Read the model definition and answer for the solid it produces. Units are mm, in the model's axes. Face numbers are marked on the shaded views. A direction names the side the tool comes from. Give positions to 0.01 mm unless a question says otherwise; leave off trailing zeros. Write each loop counter-clockwise with the first axis right and the second up, starting at its lowest first coordinate (ties: lowest second). Pieces come first, ordered by that corner, then holes.
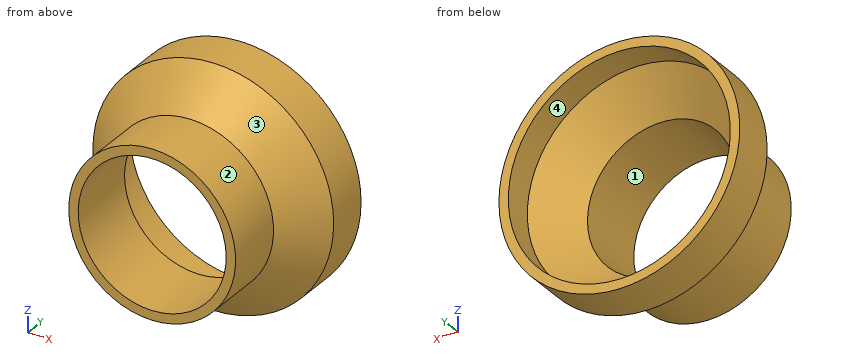
```python
from build123d import *

# Parameters (mm, degrees)
SKETCH1_R           = 15.748
SKETCH1_R_2         = 13.97
BOSS_EXTRUDE1_DEPTH = 19.05
SKETCH2_R           = 22.733
SKETCH2_R_2         = 13.97
BOSS_EXTRUDE2_DEPTH = 7.62
SKETCH3_R           = 20.955
CUT_EXTRUDE1_DEPTH  = 5.08
CHAMFER1_SIZE       = 7.62
CHAMFER2_SIZE       = 7.62


with BuildPart() as part:
    # Sketch1 → Boss-Extrude1 (new body)
    with BuildSketch(Plane(origin=(0, 0, 0), x_dir=(1, 0, 0), z_dir=(0, 1, 0))):
        with Locations(Location((0, 0, 0), (0, 0, 90))):
            Circle(SKETCH1_R)
        with Locations(Location((0, 0, 0), (0, 0, 90))):
            Circle(SKETCH1_R_2, mode=Mode.SUBTRACT)
    extrude(amount=BOSS_EXTRUDE1_DEPTH)

    # Sketch2 → Boss-Extrude2 (add)
    with BuildSketch(Plane(origin=(0, 19.05, 0), x_dir=(1, 0, 0), z_dir=(0, 1, 0))):
        with Locations(Location((0, 0, 0), (0, 0, 90))):
            Circle(SKETCH2_R)
        with Locations(Location((0, 0, 0), (0, 0, 90))):
            Circle(SKETCH2_R_2, mode=Mode.SUBTRACT)
    extrude(amount=BOSS_EXTRUDE2_DEPTH)

    # Sketch3 → Cut-Extrude1 (cut)
    with BuildSketch(Plane(origin=(0, 26.67, 0), x_dir=(1, 0, 0), z_dir=(0, 1, 0))):
        with Locations(Location((0, 0, 0), (0, 0, 270))):
            Circle(SKETCH3_R)
    extrude(amount=-CUT_EXTRUDE1_DEPTH, mode=Mode.SUBTRACT)

    # Chamfer1
    # the kernel refuses this chamfer: 7.62 mm, written as the material it adds along each edge
    with BuildSketch(Plane(origin=(0, 19.05, 0), x_dir=(0, 0, -1), z_dir=(1, 0, 0))) as chamfer1_piece_1_section:
        Polygon((15.748, -CHAMFER1_SIZE), (15.748 + CHAMFER1_SIZE, 0), (15.748, 0), align=None)
    chamfer1_piece_1 = revolve(axis=Axis((0, 19.05, 0), (0, 1, 0)), mode=Mode.PRIVATE)
    chamfer1_piece_1 = chamfer1_piece_1 & Plane(origin=(0, 14.923095596, 0), x_dir=(0, 0, -1), z_dir=(0, -1, 0)) * Cylinder(22.733, 94, mode=Mode.PRIVATE)
    add(chamfer1_piece_1)

    # Chamfer2
    # the kernel refuses this chamfer: 7.62 mm, written as the material it takes off along each edge
    with BuildSketch(Plane(origin=(0, 21.59, 0), x_dir=(0, 0, -1), z_dir=(-1, 0, 0))) as chamfer2_piece_1_section:
        Polygon((13.97, CHAMFER2_SIZE), (13.97 + CHAMFER2_SIZE, 0), (13.97, 0), align=None)
    chamfer2_piece_1 = revolve(axis=Axis((0, 21.59, 0), (0, -1, 0)), mode=Mode.PRIVATE)
    chamfer2_piece_1 = chamfer2_piece_1 & Plane(origin=(0, 17.459443448, 0), x_dir=(0, 0, 1), z_dir=(0, 1, 0)) * Cylinder(20.955, 87, mode=Mode.PRIVATE)
    add(chamfer2_piece_1, mode=Mode.SUBTRACT)


solid = part.part
```
Item 1: Determine the mould class of the marked faces 1 and 2 for opening direction Z: pulls with the +Z half, pulls with the -Z half, needs draft (parallel to the pull), parting line crosses it, or undercut.
Result set:
face 1: undercut
face 2: parting line crosses it
Item 2: Each of these flat-tipped pins is pushed along its axis until it touches: pin 1 Ø6 at (y, z) = (12, 3.5) entering from +X; pin 2 Ø6 at (y, z) = (17, -4) entering from -X; pin 3 Ø2 at (y, z) = (7, -14.5) entering from -X. Where does it stop, or does it pass through?
Result set:
pin 1: stops at x = 19.04
pin 2: stops at x = -22.69
pin 3: stops at x = -8.11
Item 3: Find the intervals of material crossed by line 1 along X through (y, z) = (23.45, 0) (3 decimals); line 2 along X through (y, z) = (7, 0), in increasing order.
Result set:
line 1: x = -22.733 to -20.955, 20.955 to 22.733
line 2: x = -15.75 to -13.97, 13.97 to 15.75
Item 4: Section C-C (y = 25.25) is taken. Write down the section's boundary in (x, z) (3 decimals), and give its area (3 significant figures).
Result set:
outline: circle Ø45.466 at (0, 0); hole circle Ø41.91 at (0, 0)
area: 244 mm2
Item 5: Section B-B (x = 0) is taken. Write down the section's boundary in (y, z) (3 decimals).
Result set:
outline: (0, -15.748) - (11.43, -15.748) - (18.415, -22.733) - (26.67, -22.733) - (26.67, -20.955) - (20.955, -20.955) - (13.97, -13.97) - (0, -13.97) - close; (0, 13.97) - (13.97, 13.97) - (20.955, 20.955) - (26.67, 20.955) - (26.67, 22.733) - (18.415, 22.733) - (11.43, 15.748) - (0, 15.748) - close
Item 6: Which of the six approach directions +Z, -Z, +X, -X, +Y, -Y give full straight-line access (tool end or side, diameter ignored) to the marked faces 3 and 4?
Result set:
face 3: -Y
face 4: +Y
Item 7: Section D-D (y = 13.25) is taken. Write down the section's boundary in (x, z), and give its area (3 significant figures).
Result set:
outline: circle Ø35.14 at (0, 0); hole circle Ø27.94 at (0, 0)
area: 356 mm2
Item 8: Section A-A (z = 0) is taken. Write down the section's boundary in (x, y) (3 decimals).
Result set:
outline: (-22.733, 18.415) - (-15.748, 11.43) - (-15.748, 0) - (-13.97, 0) - (-13.97, 13.97) - (-20.955, 20.955) - (-20.955, 26.67) - (-22.733, 26.67) - close; (13.97, 0) - (15.748, 0) - (15.748, 11.43) - (22.733, 18.415) - (22.733, 26.67) - (20.955, 26.67) - (20.955, 20.955) - (13.97, 13.97) - close
